The model under review builds one solid part; all positions refer to its coordinate system, in mm. Coordinates: 2 decimals unless noted, no trailing zeros. Order: outer loops, then holes, each group sorted by start corner. A loop starts at its lowest first (then second) coordinate and runs counter-clockwise, first axis right, second up. Notation, with made-up numbers: M 8,88.5 L 39,88.5 A27 ccw 39,105.5 Z; hole C 39,-7.5 d8. An arc over 180 degrees is marked long. Write each question's results on one line, items separated by ' | '.
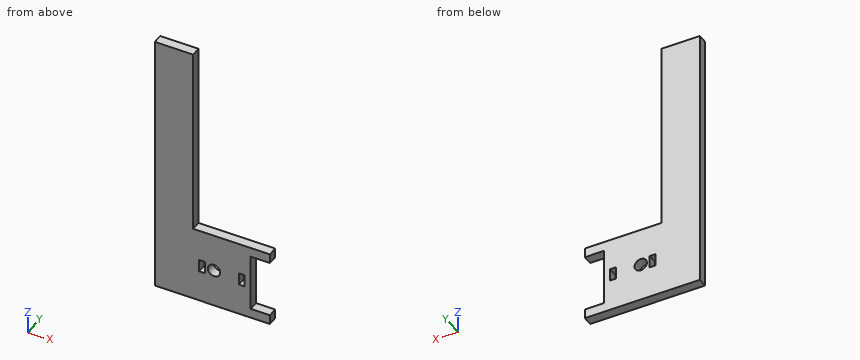
from build123d import *

# Parameters (mm, degrees)
SKETCH1_R               = 3.25
BOSS_EXTRUDE1_DEPTH     = 5
SKETCH3_W               = 20
SKETCH3_H               = 140
BOSS_EXTRUDE2_DEPTH     = 5
SKETCH4_W               = 3
SKETCH4_H               = 6.5
CUT_EXTRUDE1_DEPTH      = 1
CUT_EXTRUDE1_DEPTH_BACK = 6


with BuildPart() as part:
    # Sketch1 → Boss-Extrude1 (new body)
    with BuildSketch(Plane(origin=(0, 0, 0), x_dir=(1, 0, 0), z_dir=(0, 1, 0))):
        Polygon((-20, -15), (-30, -15), (-30, 15), (-20, 15), (-20, 20), (-60, 20), (-60, -20), (-20, -20), align=None)
        with Locations((-49.15, 0)):
            Circle(SKETCH1_R, mode=Mode.SUBTRACT)
    extrude(amount=BOSS_EXTRUDE1_DEPTH)

    # Sketch3 → Boss-Extrude2 (add)
    with BuildSketch(Plane(origin=(0, 0, 0), x_dir=(1, 0, 0), z_dir=(0, 1, 0))):
        with Locations((-70, -50)):
            Rectangle(SKETCH3_W, SKETCH3_H)
    extrude(amount=BOSS_EXTRUDE2_DEPTH)

    # Sketch4 → Cut-Extrude1 (cut, two sides)
    with BuildSketch(Plane(origin=(0, 5, 0), x_dir=(1, 0, 0), z_dir=(0, 1, 0))) as cut_extrude1_sk:
        with Locations((-34.65, 0)):
            Rectangle(SKETCH4_W, SKETCH4_H)
        with Locations((-55.35, 0)):
            Rectangle(SKETCH4_W, SKETCH4_H)
    extrude(amount=CUT_EXTRUDE1_DEPTH, mode=Mode.SUBTRACT)
    extrude(cut_extrude1_sk.sketch, amount=-CUT_EXTRUDE1_DEPTH_BACK, mode=Mode.SUBTRACT)


solid = part.part
1) To check wall thickness, follow line 1 along X through (y, z) = (1.45, 0); line 2 along Z through (x, y) = (-49.15, 2.05); line 3 along X through (y, z) = (1.1, -1). State the ranges of each line that lie inside material, in increasing order.
Solutions:
line 1: -80 to -56.85, -53.85 to -52.4, -45.9 to -36.15, -33.15 to -30 | line 2: -20 to -3.25, 3.25 to 20 | line 3: -80 to -56.85, -53.85 to -52.24, -46.06 to -36.15, -33.15 to -30
2) For pin 1 (2.5 mm diameter, centred on y = 1.5, z = -5.5, fed in from +X); pin 2 (1.5 mm diameter, centred on x = -24, y = 3.5, fed in from +Z); pin 3 (1 mm diameter, centred on y = 1, z = 54, fed in from +X), all flat-tipped, find the tip position at first contact; note any pin that passes through.
Solutions:
pin 1: x = -30 | pin 2: z = 20 | pin 3: x = -60
3) Take a section at D-D on z = 26. State the section outline as (x, y) points.
Solutions:
outline: M -80,0 L -60,0 L -60,5 L -80,5 Z
4) Take a section at B-B on x = -49.15. State the section outline as (y, z) points, plus the area to 4 significant figures.
Solutions:
outline: M 0,-20 L 5,-20 L 5,-3.25 L 0,-3.25 Z; M 0,3.25 L 5,3.25 L 5,20 L 0,20 Z | area: 167.5 mm2
5) Take a section at A-A on y = 3.3. State the section outline as (x, z) points, plus the area to 3 significant figures.
Solutions:
outline: M -80,-20 L -20,-20 L -20,-15 L -30,-15 L -30,15 L -20,15 L -20,20 L -60,20 L -60,120 L -80,120 Z; hole M -56.85,-3.25 L -53.85,-3.25 L -53.85,3.25 L -56.85,3.25 Z; hole C -49.15,0 d6.5; hole M -36.15,-3.25 L -33.15,-3.25 L -33.15,3.25 L -36.15,3.25 Z | area: 4,030 mm2
6) Take a section at C-C on z = 0. State the section outline as (x, y) points, plus the area to 4 significant figures.
Solutions:
outline: M -80,0 L -56.85,0 L -56.85,5 L -80,5 Z; M -53.85,0 L -52.4,0 L -52.4,5 L -53.85,5 Z; M -45.9,0 L -36.15,0 L -36.15,5 L -45.9,5 Z; M -33.15,0 L -30,0 L -30,5 L -33.15,5 Z | area: 187.5 mm2
